```python
from build123d import *

# Parameters (mm, degrees)
F2_DEPTH  = 23.8
F2_FACE_W = 11.670614
F2_FACE_H = 23.8
F1_R      = 2.15
F3_DEPTH  = 25
F0_R      = 2.15
F4_DEPTH  = 12
F5_DEPTH  = 12


with BuildPart() as f2:
    # F0 (on Top) → F2 (new body)
    with BuildSketch(Plane.XY):
        Polygon((-27.997939, -6.107914), (-28.312882, -16.618271), (-15.182475, -10.918183), (-8.610408, -6.107914), (-18.446828, -6.107914), (-18.446828, -10.508162), (-23.616951, -12.177606), (-25.576867, -6.107914), align=None)
        Polygon((-8.610408, -6.107914), (-15.182475, -10.918183), (-3.116295, -10.918183), (-3.116295, -6.107914), align=None)
        Polygon((-39.983496, -6.107914), (-39.983496, -16.618271), (-28.312882, -16.618271), (-27.997939, -6.107914), align=None)
    extrude(amount=F2_DEPTH)

    # F2_face (on face) + F1 (on Front) → F3 (cut)
    with BuildSketch(Plane(origin=(-34.148189, -16.618271, 11.9), x_dir=(1, 0, 0), z_dir=(0, -1, 0))):
        Rectangle(F2_FACE_W, F2_FACE_H)
    with BuildSketch(Plane.XZ):
        with Locations((-32.747678, 18.5)):
            Circle(F1_R)
        with Locations((-8.747678, 18.5)):
            Circle(F1_R)
    extrude(amount=F3_DEPTH, mode=Mode.SUBTRACT)

    # F0 (on Top) → F4 (join)
    with BuildSketch(Plane.XY):
        Polygon((6.790542, 7.431474), (-27.997939, -6.107914), (-25.576867, -6.107914), (-18.446828, -6.107914), (-8.610408, -6.107914), (-8.610408, -4.192226), (11.700466, 3.712598), (15.768237, 0), (25.596975, 2.855423), (21.576397, 13.186007), (12.574072, 7.844407), align=None)
        with Locations((18.730204, 6.14762)):
            Circle(F0_R, mode=Mode.SUBTRACT)
        Polygon((-18.446828, -6.107914), (-25.576867, -6.107914), (-23.616951, -12.177606), (-18.446828, -10.508162), align=None)
        with Locations((-21.747678, -8.362398)):
            Circle(F0_R, mode=Mode.SUBTRACT)
    extrude(amount=F4_DEPTH)

    # F0 (on Top) → F5 (cut)
    with BuildSketch(Plane.XY):
        Polygon((-8.610408, -6.107914), (-15.182475, -10.918183), (-3.116295, -10.918183), (-3.116295, -6.107914), align=None)
    extrude(amount=F5_DEPTH, mode=Mode.SUBTRACT)


solid = f2.part
```
The listing builds one solid part. Answer for the finished solid, in the listing's coordinates (mm). A direction names the side the tool comes from. Coordinates: 2 decimals unless noted, no trailing zeros. Loops run counter-clockwise (first coordinate to the right, second up) from the corner with the lowest first, then second, coordinate; pieces in that order, holes last. Notation, with made-up numbers: M 88.5,42.25 L 94.5,42.25 A27 ccw 94.5,65.25 Z; hole C 78.25,-4 d4. An arc over 180 degrees is marked long. Answer as CSV lines item,"result". Start each with the question number.
(1) Given pin 1 (1.5 mm diameter, centred on y = -5.5, z = 7, fed in from +X); pin 2 (4 mm diameter, centred on y = -7.5, z = 20.5, fed in from +X); pin 3 (5.5 mm diameter, centred on x = -8.75, z = 18.5, fed in from +Y), each flat-ended and moving along its own axis, determine where each tip first touches the part or whether it passes through.
(2) The part is cut by section C-C (x = -32). Give the vertices of the cut face in (y, z).
(3) The part is cut by section B-B (z = 3). Give the vertices of the cut face in (x, y).
(4) For faces 4 (the flat face through (-8, -9, 12)), 5 (the flat face through (-34, -16.618, 12)), 6 (the flat face through (-34, -6.108, 12)), 7 (the flat face through (20.614, 1.408, 5.916)), 8 (the flat face through (-18.447, -8, 18)), determine the directions among +Z, -Z, +X, -X, +Y, -Y from which every point of the face is accessible in a straight line to the end or side of a thin tool.
(5) The mould has two halves that part along X. Classify faces 1 (the flat face through (-11.85, -8.48, 5.92)), 2 (the cylindrical face through (-34.45, -11.29, 17.19)), 3 (the flat face through (17.138, 10.553, 5.916)): pulls with the +X half, pulls with the -X half, needs draft (parallel to the pull), parting line crosses it, or undercut.
(6) The part is cut by section D-D (z = 21.5). Give the vertices of the cut face in (x, y), and give its area (3 significant figures).
(7) The part is cut by section A-A (z = 18.5). Give the vertices of the cut face in (x, y).
(8) Find the intervals of material crossed by L1, parallel to X at y = -7.9, z = 18.5; L2, parallel to X at y = -8.9, z = 18.5; L3, parallel to Z at x = 20.5, y = 11.75, in increasing order. Write a range as [from, to].
Determined:
1,pin 1,"x = -8.61"
1,pin 2,"x = -3.12"
1,pin 3,"y = -6.11"
2,outline,"M -16.62,0 L -6.11,0 L -6.11,16.48 L -16.62,16.48 Z; M -16.62,20.52 L -6.11,20.52 L -6.11,23.8 L -16.62,23.8 Z"
3,outline,"M -39.98,-16.62 L -28.31,-16.62 L -15.18,-10.92 L -8.61,-6.11 L -8.61,-4.19 L 11.7,3.71 L 15.77,0 L 25.6,2.86 L 21.58,13.19 L 12.57,7.84 L 6.79,7.43 L -28,-6.11 L -39.98,-6.11 Z; hole C -21.75,-8.36 d4.3; hole C 18.73,6.15 d4.3"
4,face 4,"-Z, +X, -Y"
4,face 5,"+Z, -Z, +X, -X, -Y"
4,face 6,"+Z, -X, +Y"
4,face 7,"+Z, -Z, +X, -Y"
4,face 8,"+Z, +Y"
5,face 1,"pulls with the +X half"
5,face 2,"undercut"
5,face 3,"pulls with the -X half"
6,outline,"M -39.98,-16.62 L -28.31,-16.62 L -15.18,-10.92 L -3.12,-10.92 L -3.12,-6.11 L -18.45,-6.11 L -18.45,-10.51 L -23.62,-12.18 L -25.58,-6.11 L -39.98,-6.11 Z"
6,area,"248 mm2"
7,outline,"M -39.98,-16.62 L -34.9,-16.62 L -34.9,-6.11 L -39.98,-6.11 Z; M -30.6,-16.62 L -28.31,-16.62 L -15.18,-10.92 L -10.9,-10.92 L -10.9,-6.11 L -18.45,-6.11 L -18.45,-10.51 L -23.62,-12.18 L -25.58,-6.11 L -30.6,-6.11 Z; M -6.6,-10.92 L -3.12,-10.92 L -3.12,-6.11 L -6.6,-6.11 Z"
8,L1,"[-39.98, -34.9], [-30.6, -25], [-18.45, -10.9], [-6.6, -3.12]"
8,L2,"[-39.98, -34.9], [-30.6, -24.68], [-18.45, -10.9], [-6.6, -3.12]"
8,L3,"[0, 12]"
